Design review of the part built by this model. Coordinates are the model's own, in mm. A direction names the side the tool comes from. Coordinates: 2 decimals unless noted, no trailing zeros. Loops run counter-clockwise (first coordinate to the right, second up) from the corner with the lowest first, then second, coordinate; pieces in that order, holes last. Notation, with made-up numbers: M -8.5,44 L 20.5,44 A25 ccw 20.5,68 Z; hole C -24,83.5 d8. An arc over 180 degrees is marked long. Answer as a JSON object with one key per item and string values. Group by question number.
1. Consider section D-D (y = 0). State the section outline as (x, z) points (3 decimals).
2. Consider section C-C (x = 0.25). State the section outline as (y, z) points, then the cut area to 3 significant figures.
3. Insertion check: pin 1 (1.5 mm diameter, centred on x = -15.5, y = 0, fed in from +Z); pin 2 (5 mm diameter, centred on x = -1.5, z = 7, fed in from +Y); pin 3 (3.5 mm diameter, centred on x = -11.5, y = -2, fed in from +Z). Each pin has a flat end and moves straight along its axis. Give the tip position at first contact, or say it passes through.
4. To check wall thickness, follow probe 1 along Y at (x, z) = (0, 4) (3 decimals); probe 2 along Z at (x, y) = (-18, -3.5); probe 3 along Y at (x, z) = (0, 1.5) (3 decimals). State the ranges of each line that lie inside material, in increasing order.
5. Consider section B-B (y = 3.5). State the section outline as (x, z) points.
6. Draft analysis for pull direction Y (two halves, no side actions). For faces 4 (the flat face through (-11.3, 6, 1.5)), 5 (the cylindrical face through (0.808, -0.335, 2.859)), 6 (the flat face through (-18, 0, 11.8)), state which applies: +Y half, -Y half, draft (parallel to the pull), parting line (faces both ways), or undercut.
7. Consider section A-A (z = 3). State the section outline as (x, y) points (3 decimals), then the cut area to 3 significant figures.
8. Machinability: for faces 1 (the flat face through (-11, 0.9, 4)), 2 (the flat face through (-11, -0.9, 4)), 3 (the flat face through (-9.817, -0.013, 4.335)), which of the approach directions +Z, -Z, +X, -X, +Y, -Y give a long, thin tool a straight path to every point of the face, cutting with its end or side? Answer none if there is none.
from build123d import *

# Parameters (mm, degrees)
SKETCH_R        = 0.875
PAD_DEPTH       = 1.8
SKETCH001_W     = 1.8
SKETCH001_H     = 12
PAD001_DEPTH    = 10
SKETCH002_R     = 1
POCKET_DEPTH    = 1.801
SKETCH003_W     = 13.757845
SKETCH003_H     = 1.8
PAD002_DEPTH    = 5
POCKET001_DEPTH = 1.8
SKETCH005_R     = 1.9
SKETCH005_R_2   = 0.875
PAD003_DEPTH    = 4


with BuildPart() as part:
    # Sketch → Pad (new body)
    with BuildSketch(Plane.XY):
        Polygon((-18.4, 6), (2, 6), (2, 0), (2, -6), (-18.4, -6), align=None)
        Circle(SKETCH_R, mode=Mode.SUBTRACT)
    extrude(amount=PAD_DEPTH)

    # Sketch001 → Pad001 (new body)
    with BuildSketch(Plane.XY.offset(1.8)):
        with Locations((-17.5, 0)):
            Rectangle(SKETCH001_W, SKETCH001_H)
    extrude(amount=PAD001_DEPTH)

    # Sketch002 → Pocket (cut, through all)
    with BuildSketch(Plane.YZ.offset(-16.6)):
        with Locations((-3.5, 6.8)):
            Circle(SKETCH002_R)
        with Locations((3.5, 6.8)):
            Circle(SKETCH002_R)
    extrude(amount=-POCKET_DEPTH, mode=Mode.SUBTRACT)

    # Sketch003 → Pad002 (new body)
    with BuildSketch(Plane.XY.offset(1.8)):
        with Locations((-9.7210775, 0)):
            Rectangle(SKETCH003_W, SKETCH003_H)
    extrude(amount=PAD002_DEPTH)

    # Sketch004 → Pocket001 (cut)
    with BuildSketch(Plane.XZ.offset(0.9)):
        Polygon((-16.6, 6.8), (-2.842155, 1.8), (-2.842155, 6.8), align=None)
    extrude(amount=-POCKET001_DEPTH, mode=Mode.SUBTRACT)

    # Sketch005 → Pad003 (new body)
    with BuildSketch(Plane.XY.offset(1.8)):
        Circle(SKETCH005_R)
        Circle(SKETCH005_R_2, mode=Mode.SUBTRACT)
    extrude(amount=PAD003_DEPTH)


solid = part.part
Findings below:
{
 "1": {"outline": "M -18.4,0 L -0.875,0 L -0.875,5.8 L -1.9,5.8 L -1.9,1.8 L -2.842,1.8 L -16.6,6.8 L -16.6,11.8 L -18.4,11.8 Z; M 0.875,0 L 2,0 L 2,1.8 L 1.9,1.8 L 1.9,5.8 L 0.875,5.8 Z"},
 "2": {"outline": "M -6,0 L -0.84,0 L -0.84,5.8 L -1.88,5.8 L -1.88,1.8 L -6,1.8 Z; M 0.84,0 L 6,0 L 6,1.8 L 1.88,1.8 L 1.88,5.8 L 0.84,5.8 Z", "area": "26.9 mm^2"},
 "3": {"pin 1": "stops at z = 6.67", "pin 2": "stops at y = 1.9", "pin 3": "stops at z = 5.44"},
 "4": {"probe 1": "y = -1.9 to -0.875, 0.875 to 1.9", "probe 2": "z = 0 to 5.8, 7.8 to 11.8", "probe 3": "y = -6 to -0.875, 0.875 to 6"},
 "5": {"outline": "M -18.4,0 L 2,0 L 2,1.8 L -16.6,1.8 L -16.6,5.8 L -18.4,5.8 Z; M -18.4,7.8 L -16.6,7.8 L -16.6,11.8 L -18.4,11.8 Z"},
 "6": {"face 4": "+Y half", "face 5": "undercut", "face 6": "draft"},
 "7": {"outline": "M -18.4,-6 L -16.6,-6 L -16.6,-0.9 L -6.144,-0.9 L -6.144,0.9 L -16.6,0.9 L -16.6,6 L -18.4,6 Z; C 0,0 d3.8; hole C 0,0 d1.75", "area": "49.4 mm^2"},
 "8": {"face 1": "+Z, +Y", "face 2": "+Z, -Y", "face 3": "+Z, +Y, -Y"}
}
